from build123d import *

# Parameters (mm, degrees)
BOSS_EXTRUDE1_DEPTH = 3
CUT_EXTRUDE1_DEPTH  = 10
SKETCH3_W           = 194
SKETCH3_H           = 3
BOSS_EXTRUDE2_DEPTH = 32.11
SKETCH4_W           = 30
SKETCH4_H           = 18
CUT_EXTRUDE2_DEPTH  = 22
FILLET1_R           = 5
FILLET2_R           = 5


with BuildPart() as part:
    # Sketch1 → Boss-Extrude1 (new body)
    with BuildSketch(Plane.XY):
        Polygon((100, -2.5), (97, -2.5), (97, 7.5), (100, 7.5), (100, 17.5), (97, 17.5), (97, 27.5), (100, 27.5), (100, 37.5), (97, 37.5), (97, 47.5), (100, 47.5), (100, 57.5), (97, 57.5), (-97, 57.5), (-100, 57.5), (-100, 47.5), (-97, 47.5), (-97, 37.5), (-100, 37.5), (-100, 27.5), (-97, 27.5), (-97, 17.5), (-100, 17.5), (-100, 7.5), (-97, 7.5), (-97, -2.5), (-100, -2.5), (-100, -25.5), (-97, -25.5), (-82.5, -25.5), (-82.5, -28.5), (-67.5, -28.5), (-67.5, -25.5), (-52.5, -25.5), (-52.5, -28.5), (-37.5, -28.5), (-37.5, -25.5), (-22.5, -25.5), (-22.5, -28.5), (-7.5, -28.5), (-7.5, -25.5), (0, -25.5), (7.5, -25.5), (7.5, -28.5), (22.5, -28.5), (22.5, -25.5), (30, -25.5), (37.5, -25.5), (37.5, -28.5), (52.5, -28.5), (52.5, -25.5), (60, -25.5), (67.5, -25.5), (67.5, -28.5), (82.5, -28.5), (82.5, -25.5), (97, -25.5), (100, -25.5), align=None)
    extrude(amount=BOSS_EXTRUDE1_DEPTH)

    # Sketch2 → Cut-Extrude1 (cut)
    with BuildSketch(Plane.XY.offset(3)):
        with BuildLine():
            Line((55, 22.5), (55, 37.5))
            ThreePointArc((55, 37.5), (68, 50.5), (81, 37.5))
            Line((81, 37.5), (81, 22.5))
            ThreePointArc((81, 22.5), (68, 9.5), (55, 22.5))
        make_face()
    extrude(amount=-CUT_EXTRUDE1_DEPTH, mode=Mode.SUBTRACT)

    # Sketch3 → Boss-Extrude2 (add)
    with BuildSketch(Plane.XZ.offset(28.5)):
        with Locations((0, 1.5)):
            Rectangle(SKETCH3_W, SKETCH3_H)
    extrude(amount=BOSS_EXTRUDE2_DEPTH)

    # Sketch4 → Cut-Extrude2 (cut)
    with BuildSketch(Plane.XY.offset(3)):
        with Locations((0, -51.61)):
            Rectangle(SKETCH4_W, SKETCH4_H)
    extrude(amount=-CUT_EXTRUDE2_DEPTH, mode=Mode.SUBTRACT)

    # Fillet1
    fillet1_edges = [part.edges().sort_by_distance(p)[0] for p in [
        (15, -60.61, 1.5),
        (-15, -60.61, 1.5),
    ]]
    fillet(fillet1_edges, radius=FILLET1_R)

    # Fillet2
    fillet2_edges = [part.edges().sort_by_distance(p)[0] for p in [
        (-15, -42.61, 1.5),
        (15, -42.61, 1.5),
    ]]
    fillet(fillet2_edges, radius=FILLET2_R)


solid = part.part
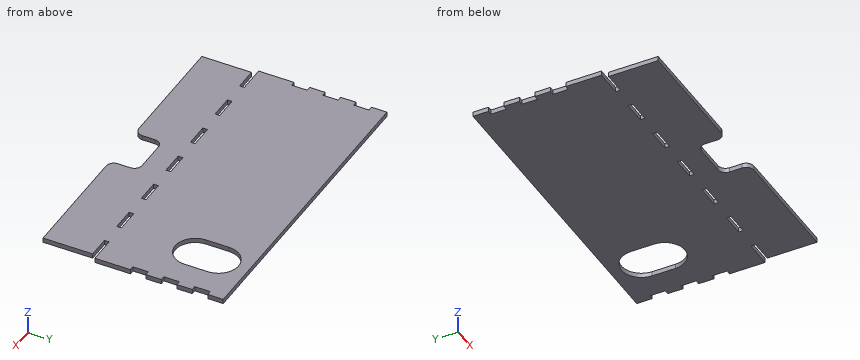
Verification items for the finished model (mm, model axes). Give positions to 0.01 mm unless a question says otherwise; leave off trailing zeros. Loops run counter-clockwise (first coordinate to the right, second up) from the corner with the lowest first, then second, coordinate; pieces in that order, holes last. Notation, with made-up numbers: (-39, 75.5) - (7, 75.5) arc R16 ccw to (7, 96.5) - close; hole circle Ø10 at (74, 89.5). An arc over 180 degrees is marked (long way). Write item = value, one per line. Start each with the question number.
Q1. Cross-section at A-A, the plane y = 25.5. Enter the section's corners in (x, z).
Q2. Cross-section at C-C, the plane z = 0.7. State how many separate pieces and enclosed holes the cut face has, and give its area (3 significant figures).
Q3. Depth check by flat-ended pin: P1, Ø1.5, axis at x = -4, z = 2, coming from the -Y side; P2, Ø0.9, axis at y = -52, z = 1, coming from the +X side; P3, Ø1.5, axis at y = -27.5, z = 2, coming from the +X side. Enter the tip coordinate at first touch or a pass-through.
Q4. Cross-section at D-D, the plane y = -31.5. Enter the section's corners in (x, z).
Q5. Cross-section at B-B, the plane x = -33. Enter the section's corners in (y, z), and give its area (3 significant figures).
Q6. Thickness scan on line 1 (X direction, y = 37, z = 0.8); line 2 (Y direction, x = 5, z = 0.75); line 3 (Y direction, x = 87, z = 1.65). Record the ranges inside material, lowest first.
Answer key:
q1.outline = (-97, 0) - (55, 0) - (55, 3) - (-97, 3) - close; (81, 0) - (97, 0) - (97, 3) - (81, 3) - close
q2.separate_pieces = 1
q2.enclosed_holes = 6
q2.area = 21,500 mm^2
q3.P1 = -42.61
q3.P2 = 97
q3.P3 = 82.5
q4.outline = (-97, 0) - (97, 0) - (97, 3) - (-97, 3) - close
q5.outline = (-60.61, 0) - (-28.5, 0) - (-28.5, 3) - (-60.61, 3) - close; (-25.5, 0) - (57.5, 0) - (57.5, 3) - (-25.5, 3) - close
q5.area = 345 mm^2
q6.line_1 = -100 to 55, 81 to 100
q6.line_2 = -42.61 to -28.5, -25.5 to 57.5
q6.line_3 = -60.61 to -28.5, -25.5 to 57.5
